Can you work these out from the model? Positions are in its coordinate system, mm. A direction names the side the tool comes from. Round coordinates to 2 decimals unless told otherwise and drop trailing zeros. Loops run counter-clockwise (first coordinate to the right, second up) from the corner with the lowest first, then second, coordinate; pieces in that order, holes last. Notation, with made-up numbers: (21.5, 79.25) -> (49.5, 79.25) arc R27 cw to (49.5, 111.25) -> close; hole circle Ø4 at (25.25, -9). An arc over 180 degrees is marked (long way). Use a Markdown table: item, result.
from build123d import *

# Parameters (mm, degrees)
F0_R          = 3
F1_DEPTH      = 3.6
F3_DEPTH      = 3.6
F5_DEPTH      = 3.6
F6_R          = 4
F7_DEPTH      = 7.201
F7_DEPTH_BACK = 3.601


with BuildPart() as f1:
    # F0 (on Front) → F1 (new body)
    with BuildSketch(Plane.XZ):
        with BuildLine():
            Line((22, 12), (0, 12))
            ThreePointArc((0, 12), (-6, 6), (0, 0))
            Line((0, 0), (22, 0))
            ThreePointArc((22, 0), (28, 6), (22, 12))
        make_face()
        with Locations((0, 6)):
            Circle(F0_R, mode=Mode.SUBTRACT)
    extrude(amount=F1_DEPTH)

    # F2 (on Front) → F3 (join)
    with BuildSketch(Plane.XZ):
        with BuildLine():
            Line((46, 12), (22, 12))
            ThreePointArc((22, 12), (16, 6), (22, 0))
            Line((22, 0), (46, 0))
            ThreePointArc((46, 0), (52, 6), (46, 12))
        make_face()
    extrude(amount=-F3_DEPTH)

    # F4 (on face) → F5 (join)
    with BuildSketch(Plane.XZ.offset(3.6)):
        with BuildLine():
            Line((46, 12), (22, 12))
            ThreePointArc((22, 12), (16, 6), (22, 0))
            Line((22, 0), (46, 0))
            ThreePointArc((46, 0), (52, 6), (46, 12))
        make_face()
    extrude(amount=F5_DEPTH)

    # F6 (on face) → F7 (cut, two sides)
    with BuildSketch(Plane.XZ) as f7_sk:
        with Locations((46, 6)):
            Circle(F6_R)
    extrude(amount=F7_DEPTH, mode=Mode.SUBTRACT)
    extrude(f7_sk.sketch, amount=-F7_DEPTH_BACK, mode=Mode.SUBTRACT)


solid = f1.part
1. I need wall thicknesses on line 1 (Y direction, x = 32, z = 8.5); line 2 (Z direction, x = 46, y = -4.8); line 3 (Y direction, x = 4, z = 4.25). Which ranges of each line are inside material? Lowest first, please.
Answer sheet:
| item | result |
|---|---|
| line 1 | y = -7.2 to -3.6, 0 to 3.6 |
| line 2 | z = 0 to 2, 10 to 12 |
| line 3 | y = -3.6 to 0 |
2. If we mould it in two halves opening along Y, with no side actions, what happens to faces 1 (the flat face through (11, -2, 12)), 2 (the flat face through (34, -7.2, 6)), 3 (the flat face through (37, 0, 6))? For each: +Y half, -Y half, draft (parallel to the pull), parting line (faces both ways), or undercut.
Answer sheet:
| item | result |
|---|---|
| face 1 | draft |
| face 2 | -Y half |
| face 3 | undercut |
3. I want a section at C-C (z = 6). Please give me the cut outline in (x, y), plus the area to 3 significant figures.
Answer sheet:
| item | result |
|---|---|
| outline | (-6, -3.6) -> (-3, -3.6) -> (-3, 0) -> (-6, 0) -> close; (3, -3.6) -> (16, -3.6) -> (16, -7.2) -> (42, -7.2) -> (42, -3.6) -> (28, -3.6) -> (28, 0) -> (42, 0) -> (42, 3.6) -> (16, 3.6) -> (16, 0) -> (3, 0) -> close; (50, -7.2) -> (52, -7.2) -> (52, -3.6) -> (50, -3.6) -> close; (50, 0) -> (52, 0) -> (52, 3.6) -> (50, 3.6) -> close |
| area | 302 mm² |
4. Which directions (+Z, -Z, +X, -X, +Y, -Y) give clear straight access to the entire face, cutting with the end or side of a thin tool? Please do faces 4 (the flat face through (11, -2, 0)), 5 (the cylindrical face through (28, -2, 6)), 6 (the cylindrical face through (16, 2, 6)).
Answer sheet:
| item | result |
|---|---|
| face 4 | -Z, +X, -X, +Y, -Y |
| face 5 | +X |
| face 6 | -X, +Y |
5. I want a section at B-B (x = 35.5). Please give me the cut outline in (y, z), plus the area to 3 significant figures.
Answer sheet:
| item | result |
|---|---|
| outline | (-7.2, 0) -> (-3.6, 0) -> (-3.6, 12) -> (-7.2, 12) -> close; (0, 0) -> (3.6, 0) -> (3.6, 12) -> (0, 12) -> close |
| area | 86.4 mm² |
6. I want a section at D-D (z = 9.5). Please give me the cut outline in (x, y).
Answer sheet:
| item | result |
|---|---|
| outline | (-4.87, -3.6) -> (17.13, -3.6) -> (17.13, -7.2) -> (44.06, -7.2) -> (44.06, -3.6) -> (26.87, -3.6) -> (26.87, 0) -> (44.06, 0) -> (44.06, 3.6) -> (17.13, 3.6) -> (17.13, 0) -> (-4.87, 0) -> close; (47.94, -7.2) -> (50.87, -7.2) -> (50.87, -3.6) -> (47.94, -3.6) -> close; (47.94, 0) -> (50.87, 0) -> (50.87, 3.6) -> (47.94, 3.6) -> close |
7. I want a section at A-A (y = -1). Please give me the cut outline in (x, z), plus the area to 3 significant figures.
Answer sheet:
| item | result |
|---|---|
| outline | (0, 0) -> (22, 0) arc R6 ccw to (22, 12) -> (0, 12) arc R6 ccw to start; hole circle Ø6 at (0, 6) |
| area | 349 mm² |
8. Will these pins go through, and if not, where does the flat tip stop? pin 1 Ø3.5 at (x, z) = (1.5, 6.5) entering from -Y; pin 2 Ø2 at (y, z) = (1, 1.5) entering from +X.
Answer sheet:
| item | result |
|---|---|
| pin 1 | stops at y = -3.6 |
| pin 2 | stops at x = 50.87 |
